```python
from build123d import *

# Parameters (mm, degrees)
SKETCH3_W                = 12.7
SKETCH3_H                = 15.875
SKETCH3_R                = 1.397
BOSS_EXTRUDE1_DEPTH      = 3.81
BOSS_EXTRUDE2_DEPTH      = 4.064
BOSS_EXTRUDE2_DEPTH_BACK = 4.064
SKETCH5_R                = 2.694076836
SKETCH6_R                = 1.27
BOSS_EXTRUDE3_DEPTH      = 1.778
BOSS_EXTRUDE4_START      = 1.778
SKETCH7_R                = 1.27
BOSS_EXTRUDE4_DEPTH      = 1.778


with BuildPart() as part:
    # Sketch3 → Boss-Extrude1 (new body)
    with BuildSketch(Plane(origin=(0, 0, 0), x_dir=(1, 0, 0), z_dir=(0, 1, 0))):
        with Locations((6.35, 7.9375)):
            Rectangle(SKETCH3_W, SKETCH3_H)
        with Locations(Location((3.048, 3.81, 0), (0, 0, 90))):
            Circle(SKETCH3_R, mode=Mode.SUBTRACT)
        with Locations(Location((3.048, 12.065, 0), (0, 0, 90))):
            Circle(SKETCH3_R, mode=Mode.SUBTRACT)
    extrude(amount=BOSS_EXTRUDE1_DEPTH)

    # Sketch5 → Boss-Extrude2 (add, two sides: drawn at the far end of the back side and taken through both)
    with BuildSketch(Plane.XY.offset(-7.9375).offset(-BOSS_EXTRUDE2_DEPTH_BACK)):
        with Locations((14.605, 1.905)):
            Circle(SKETCH5_R)
    extrude(amount=BOSS_EXTRUDE2_DEPTH + BOSS_EXTRUDE2_DEPTH_BACK)

    # Sketch6 → Boss-Extrude3 (add)
    with BuildSketch(Plane.XY.offset(-3.8735)):
        with Locations((14.605, 1.905)):
            Circle(SKETCH6_R)
    extrude(amount=BOSS_EXTRUDE3_DEPTH)

    # Sketch7 → Boss-Extrude4 (add)
    with BuildSketch(Plane(origin=(0, 0, -12.0015), x_dir=(-1, 0, 0), z_dir=(0, 0, -1)).offset(BOSS_EXTRUDE4_START)):
        with Locations(Location((-14.605, 1.905, 0), (0, 0, 180))):
            Circle(SKETCH7_R)
    extrude(amount=-BOSS_EXTRUDE4_DEPTH)


solid = part.part
```
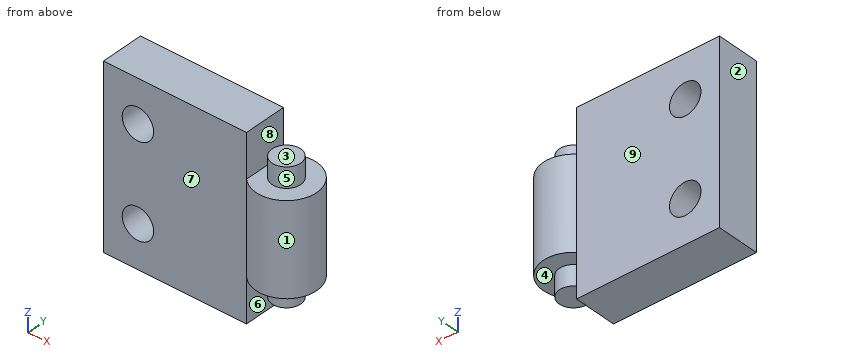
Geometry check sheet. Reference: the model listing, model coordinates, mm. Face numbers are marked on the shaded views. A direction names the side the tool comes from. Coordinates: 2 decimals unless noted, no trailing zeros. Loops run counter-clockwise (first coordinate to the right, second up) from the corner with the lowest first, then second, coordinate; pieces in that order, holes last.
Item 1: Sectioned sample at A-A, the plane y = 0.35. Record the boundary of the cut face in (x, z) (1 decimal), then the cut area to 3 significant figures.
Item 2: Go/stop test with flat-tipped pins: pin 1 Ø1.1 at (y, z) = (1, -14) entering from +X; pin 2 Ø6.5 at (x, z) = (6, -8) entering from +Y; pin 3 Ø2 at (x, y) = (14.5, 1.5) entering from -Z. Record where each tip stops, or that it passes through.
Item 3: Sectioned sample at B-B, the plane x = 7.25. Record the boundary of the cut face in (y, z) (3 decimals), then the cut area to 3 significant figures.
Item 4: Thickness scan on line 1 (X direction, y = 2.4, z = -3.81) (3 decimals); line 2 (X direction, y = 0.8, z = -3.81) (3 decimals); line 3 (Y direction, x = 5.75, z = -10.75). Record the ranges inside material, lowest first.
Item 5: Release check for a two-part mould opening along X. For the marked faces 1, 2, 3 and 4 record: released by +X, released by -X, zero draft, split by the parting line, or undercut.
Item 6: Access from +Z, -Z, +X, -X, +Y, -Y to the whole of each face (thin tool, end or side, straight path). Record for the marked faces 5, 6, 7, 8 and 9.
Check result:
1. outline: (0, -15.9) - (12.7, -15.9) - (12.7, -12) - (16.8, -12) - (16.8, -3.9) - (12.7, -3.9) - (12.7, 0) - (0, 0) - close; hole circle Ø2.8 at (3, -12.1); hole circle Ø2.8 at (3, -3.8)
1. area: 223 mm2
2. pin 1: stops at x = 15.81
2. pin 2: stops at y = 3.81
2. pin 3: stops at z = -13.78
3. outline: (0, -15.875) - (3.81, -15.875) - (3.81, 0) - (0, 0) - close
3. area: 60.5 mm2
4. line 1: x = 0 to 1.651, 4.445 to 12.7, 13.435 to 15.775
4. line 2: x = 0 to 1.651, 4.445 to 12.7, 13.979 to 15.231
4. line 3: y = 0 to 3.81
5. face 1: split by the parting line
5. face 2: released by -X
5. face 3: zero draft
5. face 4: undercut
6. face 5: +Z
6. face 6: -Z, +Y, -Y
6. face 7: +Z, -Z, -X, -Y
6. face 8: +Z, +Y, -Y
6. face 9: +Z, -Z, -X, +Y
